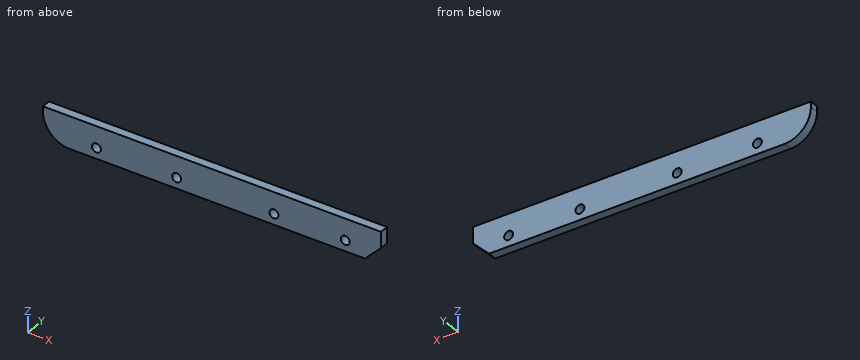
```python
from build123d import *

# Parameters (mm, degrees)
F0_W     = 189.6
F0_H     = 18
F0_R     = 2.5
F1_DEPTH = 5
F3_DEPTH = 25
F4_R     = 15


with BuildPart() as f1:
    # F0 (on Front) → F1 (new body)
    with BuildSketch(Plane.XZ):
        Rectangle(F0_W, F0_H)
        with Locations((-64.8, -3)):
            Circle(F0_R, mode=Mode.SUBTRACT)
        with Locations((-19.8, -3)):
            Circle(F0_R, mode=Mode.SUBTRACT)
        with Locations((34.8, -3)):
            Circle(F0_R, mode=Mode.SUBTRACT)
        with Locations((74.8, -3)):
            Circle(F0_R, mode=Mode.SUBTRACT)
    extrude(amount=F1_DEPTH)

    # F2 (on face) → F3 (cut)
    with BuildSketch(Plane.XZ.offset(5)):
        Polygon((94.8, -9), (94.8, 0), (85.8, -9), align=None)
    extrude(amount=-F3_DEPTH, mode=Mode.SUBTRACT)

    # F4
    f4_edges = [f1.edges().sort_by_distance(p)[0] for p in [
        (-94.8, -2.5, -9),
    ]]
    fillet(f4_edges, radius=F4_R)


solid = f1.part
```
Work out the finished part from the listing and answer in its coordinate system (mm). Coordinates: 2 decimals unless noted, no trailing zeros. Loops run counter-clockwise (first coordinate to the right, second up) from the corner with the lowest first, then second, coordinate; pieces in that order, holes last. Notation, with made-up numbers: M 68.25,-5 L 102.25,-5 A11 ccw 102.25,-1 Z; hole C 79.25,83 d4. An arc over 180 degrees is marked long. Use CSV: the item, a comma, the result in double quotes. Start each with the question number.
(1) Find section B-B, the plane z = -3. Give the vertices of the cut face in (x, y).
(2) Consider line 1 (Z direction, x = 34.8, y = -3.4); line 2 (X direction, y = -2.15, z = -2); line 3 (X direction, y = -3.5, z = -2.75). Determine where each line is inside the solid, lowest interval first.
(3) Find section A-A, the plane x = 74.8. Give the vertices of the cut face in (y, z).
(4) Find section C-C, the plane y = -3. Give the vertices of the cut face in (x, z).
(5) Given pin 1 Ø10 at (x, z) = (-1.5, 7) entering from +Y, flat-ended and moving along its own axis, determine where the tip first touches the part or whether it passes through.
Recorded:
1,outline,"M -91.8,-5 L -67.3,-5 L -67.3,0 L -91.8,0 Z; M -62.3,-5 L -22.3,-5 L -22.3,0 L -62.3,0 Z; M -17.3,-5 L 32.3,-5 L 32.3,0 L -17.3,0 Z; M 37.3,-5 L 72.3,-5 L 72.3,0 L 37.3,0 Z; M 77.3,-5 L 91.8,-5 L 91.8,0 L 77.3,0 Z"
2,line 1,"z = -9 to -5.5, -0.5 to 9"
2,line 2,"x = -92.49 to -67.09, -62.51 to -22.09, -17.51 to 32.51, 37.09 to 72.51, 77.09 to 92.8"
2,line 3,"x = -91.98 to -67.29, -62.31 to -22.29, -17.31 to 32.31, 37.29 to 72.31, 77.29 to 92.05"
3,outline,"M -5,-9 L 0,-9 L 0,-5.5 L -5,-5.5 Z; M -5,-0.5 L 0,-0.5 L 0,9 L -5,9 Z"
4,outline,"M -94.8,6 A15 ccw -79.8,-9 L 85.8,-9 L 94.8,0 L 94.8,9 L -94.8,9 Z; hole C -64.8,-3 d5; hole C -19.8,-3 d5; hole C 34.8,-3 d5; hole C 74.8,-3 d5"
5,pin 1,"stops at y = 0"
